from build123d import *

# Parameters (mm, degrees)
SKETCH1_R           = 2.667
BOSS_EXTRUDE1_DEPTH = 3.175
CHAMFER1_SIZE       = 0.635


with BuildPart() as part:
    # Sketch1 → Boss-Extrude1 (new, symmetric)
    with BuildSketch(Plane(origin=(0, 0, 0), x_dir=(1, 0, 0), z_dir=(0, 1, 0))):
        Polygon((0, 36.83), (0, 4.445), (4.445, 4.445), (4.445, 0), (31.75, 0), align=None)
        with Locations(Location((8.89, 19.709926136, 0), (0, 0, 270))):
            Circle(SKETCH1_R, mode=Mode.SUBTRACT)
        with Locations(Location((13.97, 13.817126136, 0), (0, 0, 270))):
            Circle(SKETCH1_R, mode=Mode.SUBTRACT)
        with Locations(Location((19.05, 7.924326136, 0), (0, 0, 270))):
            Circle(SKETCH1_R, mode=Mode.SUBTRACT)
    extrude(amount=BOSS_EXTRUDE1_DEPTH, both=True)

    # Chamfer1
    chamfer1_edges = [part.edges().sort_by_distance(p)[0] for p in [
        (8.89, -3.175, -22.376926136),
        (8.89, 3.175, -22.376926136),
        (13.97, -3.175, -16.484126136),
        (13.97, 3.175, -16.484126136),
        (19.05, -3.175, -10.591326136),
        (19.05, 3.175, -10.591326136),
    ]]
    chamfer(chamfer1_edges, length=CHAMFER1_SIZE)


solid = part.part
Geometry check sheet. Reference: the model listing, model coordinates, mm. A direction names the side the tool comes from. Coordinates: 2 decimals unless noted, no trailing zeros. Write each loop counter-clockwise with the first axis right and the second up, starting at its lowest first coordinate (ties: lowest second). Pieces come first, ordered by that corner, then holes. Notation, with made-up numbers: (-38.75, 19.25) -> (6.25, 19.25) arc R15 cw to (6.25, 24.25) -> close; hole circle Ø7 at (28, 16). An arc over 180 degrees is marked (long way). One line per question, with ' | ' between items.
1. Cross-section at B-B on y = 0.5. Record the cut outline in (x, z) (3 decimals).
Answers:
outline: (0, -36.83) -> (31.75, 0) -> (4.445, 0) -> (4.445, -4.445) -> (0, -4.445) -> close; hole circle Ø5.334 at (8.89, -19.71); hole circle Ø5.334 at (13.97, -13.817); hole circle Ø5.334 at (19.05, -7.924)
2. Depth check by flat-ended pin: pin 1 Ø4.5 at (x, z) = (8.89, -19.71) entering from +Y; pin 2 Ø1.3 at (x, y) = (3, 1) entering from +Z (3 decimals); pin 3 Ø3 at (x, y) = (19.5, -1) entering from -Z; pin 4 Ø3 at (x, y) = (4.5, -0.5) entering from -Z. Enter the tip coordinate at first touch or a pass-through.
Answers:
pin 1: passes through | pin 2: stops at z = -4.445 | pin 3: stops at z = -15.95 | pin 4: stops at z = -33.35
3. Cross-section at A-A on x = 19.05. Record the cut outline in (y, z) (3 decimals).
Answers:
outline: (-3.175, -14.732) -> (3.175, -14.732) -> (3.175, -11.226) -> (2.54, -10.591) -> (-2.54, -10.591) -> (-3.175, -11.226) -> close; (-3.175, -4.622) -> (-2.54, -5.257) -> (2.54, -5.257) -> (3.175, -4.622) -> (3.175, 0) -> (-3.175, 0) -> close
4. Cross-section at D-D on z = -33.5. Record the cut outline in (x, y) (3 decimals), and give its area (3 significant figures).
Answers:
outline: (0, -3.175) -> (2.871, -3.175) -> (2.871, 3.175) -> (0, 3.175) -> close | area: 18.2 mm²
5. Cross-section at C-C on x = 8.89. Record the cut outline in (y, z) (3 decimals).
Answers:
outline: (-3.175, -26.518) -> (3.175, -26.518) -> (3.175, -23.012) -> (2.54, -22.377) -> (-2.54, -22.377) -> (-3.175, -23.012) -> close; (-3.175, -16.408) -> (-2.54, -17.043) -> (2.54, -17.043) -> (3.175, -16.408) -> (3.175, 0) -> (-3.175, 0) -> close
6. Draft check along Z on faces 3 (the cylindrical face through (11.14, -0.04, -18.28)), 4 (the cylindrical face through (11.366, -0.036, -14.395)), 5 (the flat face through (16.097, 0.044, -18.157)), 6 (the flat face through (0, 0, -21)). Enter one of: +Z half, -Z half, draft (parallel to the pull), parting line (faces both ways), or undercut.
Answers:
face 3: undercut | face 4: undercut | face 5: -Z half | face 6: draft
7. Thickness scan on probe 1 along X at (y, z) = (-2.25, -6.5); probe 2 along Z at (x, y) = (12, -1); probe 3 along X at (y, z) = (2.75, -18.5). Record the ranges inside material, lowest first. Write a range as from..to.
Answers:
probe 1: x = 0..16.8, 21.3..26.15 | probe 2: z = -22.91..-15.61, -12.02..0 | probe 3: x = 0..6.28, 11.5..15.8
8. Set-up check for faces 1 (the flat face through (2, 0, -4.445)), 2 (the flat face through (18, 0, 0)): record each of +Z, -Z, +X, -X, +Y, -Y from which the full face is reachable in a straight line by a thin tool's end or side.
Answers:
face 1: +Z, -X, +Y, -Y | face 2: +Z, +X, -X, +Y, -Y
